```python
from build123d import *

# Parameters (mm, degrees)
CROQUIS1_W              = 50.8
CROQUIS1_H              = 50.8
CROQUIS1_W_2            = 48.0568
CROQUIS1_H_2            = 48.0568
SALIENTE_EXTRUIR1_DEPTH = 300


with BuildPart() as part:
    # Croquis1 → Saliente-Extruir1 (new body)
    with BuildSketch(Plane.XY):
        with Locations((0, -80)):
            Rectangle(CROQUIS1_W, CROQUIS1_H)
        with Locations((0, -80)):
            Rectangle(CROQUIS1_W_2, CROQUIS1_H_2, mode=Mode.SUBTRACT)
    extrude(amount=SALIENTE_EXTRUIR1_DEPTH)


solid = part.part
```
Check sheet for the modelled part. Datum: model origin and axes. Units: mm. A direction names the side the tool comes from. Give positions to 0.01 mm unless a question says otherwise; leave off trailing zeros. Order: outer loops, then holes, each group sorted by start corner. A loop starts at its lowest first (then second) coordinate and runs counter-clockwise, first axis right, second up. Notation, with made-up numbers: M 45,60 L 95,60 A7 cw 95,73 Z; hole C -28,15 d2. An arc over 180 degrees is marked long. Answer in a Markdown table with one row per item.
1) Access from +Z, -Z, +X, -X, +Y, -Y to the whole of each face (thin tool, end or side, straight path). Record for faces 1 (the flat face through (0, -54.6, 148)), 2 (the flat face through (0, -104.028, 148)).
Filled sheet:
| item | result |
|---|---|
| face 1 | +Z, -Z, +X, -X, +Y |
| face 2 | +Z, -Z |
2) Cross-section at B-B, the plane x = -21.5. Enter the section's corners in (y, z).
Filled sheet:
| item | result |
|---|---|
| outline | M -105.4,0 L -104.03,0 L -104.03,300 L -105.4,300 Z; M -55.97,0 L -54.6,0 L -54.6,300 L -55.97,300 Z |
3) Release check for a two-part mould opening along X. For faces 3 (the flat face through (-24.028, -80, 148)), 4 (the flat face through (25.4, -80, 148)), 5 (the flat face through (-25.4, -80, 148)), 6 (the flat face through (0, -105.4, 148)) record: +X half, -X half, draft (parallel to the pull), parting line (faces both ways), or undercut.
Filled sheet:
| item | result |
|---|---|
| face 3 | undercut |
| face 4 | +X half |
| face 5 | -X half |
| face 6 | draft |
4) Thickness scan on L1, parallel to Y at x = -4, z = 74; L2, parallel to X at y = -75, z = 233. Record the ranges inside material, lowest first. Write a range as [from, to].
Filled sheet:
| item | result |
|---|---|
| L1 | y = [-105.4, -104.03], [-55.97, -54.6] |
| L2 | x = [-25.4, -24.03], [24.03, 25.4] |
5) Cross-section at C-C, the plane z = 26. Enter the section's corners in (x, y), plus the area to 3 significant figures.
Filled sheet:
| item | result |
|---|---|
| outline | M -25.4,-105.4 L 25.4,-105.4 L 25.4,-54.6 L -25.4,-54.6 Z; hole M -24.03,-104.03 L 24.03,-104.03 L 24.03,-55.97 L -24.03,-55.97 Z |
| area | 271 mm2 |
6) Cross-section at A-A, the plane y = -73. Enter the section's corners in (x, z), plus the area to 3 significant figures.
Filled sheet:
| item | result |
|---|---|
| outline | M -25.4,0 L -24.03,0 L -24.03,300 L -25.4,300 Z; M 24.03,0 L 25.4,0 L 25.4,300 L 24.03,300 Z |
| area | 823 mm2 |
